Read the model definition and answer for the solid it produces. Units are mm, in the model's axes. Round coordinates to 2 decimals unless told otherwise and drop trailing zeros. Order: outer loops, then holes, each group sorted by start corner. A loop starts at its lowest first (then second) coordinate and runs counter-clockwise, first axis right, second up. Notation, with made-up numbers: (12, 4) - (61, 4) arc R26 cw to (61, 42) - close; hole circle Ø1 at (75, -9.75). An arc over 180 degrees is marked (long way). Answer as a JSON object with one key per item and string values. Group by question number.
Q1. A cutting plane is placed at C-C on y = -1.1. Count the separate pieces of the cut face and the enclosed holes in it, and give its area (3 significant figures).
Q2. A cutting plane is placed at A-A on z = 6. Determine the outline of the cut face in (x, y).
Q3. A cutting plane is placed at B-B on x = 37. Determine the outline of the cut face in (y, z), and give its area (3 significant figures).
Q4. Given pin 1 Ø3.5 at (x, z) = (6, 6) entering from -Y, flat-ended and moving along its own axis, determine where the tip first touches the part or whether it passes through.
Q5. Consider line 1 (Z direction, x = 6, y = -0.8); line 2 (Z direction, x = 21.5, y = -0.8); line 3 (Z direction, x = 18, y = -0.45). Determine where each line is inside the solid, lowest interval first.
Q6. A cutting plane is placed at D-D on z = 27.5. Determine the outline of the cut face in (x, y).
```python
from build123d import *

# Parameters (mm, degrees)
F0_R     = 1.6
F1_DEPTH = 2


with BuildPart() as f1:
    # F0 (on Front) → F1 (new body)
    with BuildSketch(Plane.XZ):
        with BuildLine():
            ThreePointArc((0, 4.5), (1.318019, 1.318019), (4.5, 0))
            Line((4.5, 0), (43.5, 0))
            ThreePointArc((43.5, 0), (46.681981, 1.318019), (48, 4.5))
            Line((48, 4.5), (48, 18))
            ThreePointArc((48, 18), (35.698485, 47.698485), (6, 60))
            Line((6, 60), (4.5, 60))
            ThreePointArc((4.5, 60), (1.318019, 58.681981), (0, 55.5))
            Line((0, 55.5), (0, 4.5))
        make_face()
        with Locations((6, 6)):
            Circle(F0_R, mode=Mode.SUBTRACT)
        with Locations((18, 6)):
            Circle(F0_R, mode=Mode.SUBTRACT)
        with Locations((6, 18)):
            Circle(F0_R, mode=Mode.SUBTRACT)
        with BuildLine():
            ThreePointArc((16.4, 18), (13.353911, 25.353911), (6, 28.4))
            ThreePointArc((6, 28.4), (4.4, 30), (6, 31.6))
            ThreePointArc((6, 31.6), (15.616652, 27.616652), (19.6, 18))
            ThreePointArc((19.6, 18), (18, 16.4), (16.4, 18))
        make_face(mode=Mode.SUBTRACT)
        with Locations((30, 6)):
            Circle(F0_R, mode=Mode.SUBTRACT)
        with Locations((42, 6)):
            Circle(F0_R, mode=Mode.SUBTRACT)
        with BuildLine():
            ThreePointArc((28.4, 18), (21.839192, 33.839192), (6, 40.4))
            ThreePointArc((6, 40.4), (4.4, 42), (6, 43.6))
            ThreePointArc((6, 43.6), (24.101934, 36.101934), (31.6, 18))
            ThreePointArc((31.6, 18), (30, 16.4), (28.4, 18))
        make_face(mode=Mode.SUBTRACT)
        with BuildLine():
            ThreePointArc((40.4, 18), (30.324473, 42.324473), (6, 52.4))
            ThreePointArc((6, 52.4), (4.4, 54), (6, 55.6))
            ThreePointArc((6, 55.6), (32.587215, 44.587215), (43.6, 18))
            ThreePointArc((43.6, 18), (42, 16.4), (40.4, 18))
        make_face(mode=Mode.SUBTRACT)
    extrude(amount=F1_DEPTH)


solid = f1.part
```
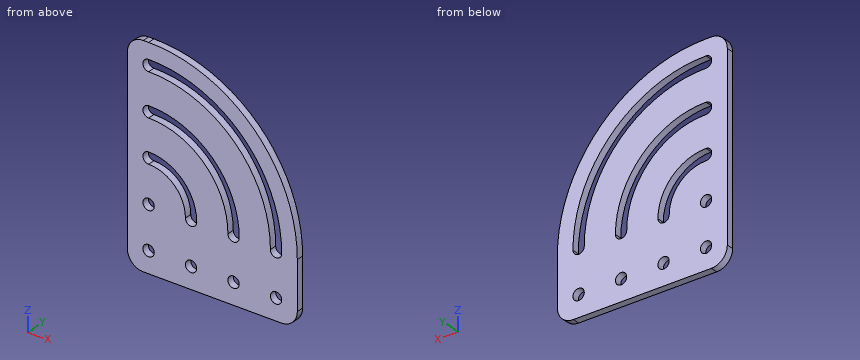
Result set:
{
 "1": {"separate pieces": "1", "enclosed holes": "8", "area": "2,060 mm²"},
 "2": {"outline": "(0, -2) - (4.4, -2) - (4.4, 0) - (0, 0) - close; (7.6, -2) - (16.4, -2) - (16.4, 0) - (7.6, 0) - close; (19.6, -2) - (28.4, -2) - (28.4, 0) - (19.6, 0) - close; (31.6, -2) - (40.4, -2) - (40.4, 0) - (31.6, 0) - close; (43.6, -2) - (48, -2) - (48, 0) - (43.6, 0) - close"},
 "3": {"outline": "(-2, 0) - (0, 0) - (0, 32.91) - (-2, 32.91) - close; (-2, 39.28) - (0, 39.28) - (0, 46.34) - (-2, 46.34) - close", "area": "79.9 mm²"},
 "4": {"pin 1": "stops at y = -2"},
 "5": {"line 1": "z = 0 to 4.4, 7.6 to 16.4, 19.6 to 28.4, 31.6 to 40.4, 43.6 to 52.4, 55.6 to 60", "line 2": "z = 0 to 34.17, 38.37 to 48.71, 52.26 to 57.04", "line 3": "z = 0 to 4.4, 7.6 to 16.4, 24.4 to 36.91, 40.61 to 50.24, 53.63 to 58.25"},
 "6": {"outline": "(0, -2) - (10.23, -2) - (10.23, 0) - (0, 0) - close; (15.73, -2) - (26.29, -2) - (26.29, 0) - (15.73, 0) - close; (29.77, -2) - (39.06, -2) - (39.06, 0) - (29.77, 0) - close; (42.38, -2) - (46.91, -2) - (46.91, 0) - (42.38, 0) - close"}
}
